Can you work these out from the model? Positions are in its coordinate system, mm. A direction names the side the tool comes from. Give positions to 0.01 mm unless a question says otherwise; leave off trailing zeros. Write each loop counter-clockwise with the first axis right and the second up, starting at its lowest first coordinate (ties: lowest second). Pieces come first, ordered by that corner, then holes. Notation, with made-up numbers: (80.25, 52) -> (91.25, 52) arc R23 cw to (91.25, 62) -> close; hole circle Ø6 at (32, 4). An arc over 180 degrees is marked (long way). Answer as CSV lines item,"result". Start each with the question number.
1. On a 3-axis mill with a long thin cutter (end or side, diameter ignored), from which of +Z, -Z, +X, -X, +Y, -Y can I reach the whole of each face in a straight line? I mean faces 1 (the face through (-3.6, 13.1, -0.5)), 2 (the face through (3.6, 13, -0.5)), 3 (the face through (4.832, 3.719, 15.463)), 4 (the face through (0.1, 18.1, -0.5)). Say none if no direction works.
2. I'm going to push flat-ended pins straight in: P1, Ø1.3, axis at x = 1, y = 17.5, coming from the +Z side; P2, Ø0.5, axis at y = 13, z = -0.5, coming from the +X side; P3, Ø8.5, axis at x = 1.5, z = 15, coming from the +Y side. Where does each tip first touch, or does it pass through?
3. If we section it at A-A on y = 27: Write out the boundary of the cut face in (x, z).
4. If we section it at C-C on z = 2: Write out the boundary of the cut face in (x, y).
5. I need wall thicknesses on line 1 (X direction, y = 2.4, z = 18); line 2 (X direction, y = 6, z = 12); line 3 (Y direction, x = 0, z = 3.35). Which ranges of each line are inside material? Lowest first, please. Write a range as [from, to].
6. If we mould it in two halves opening along Z, with no side actions, what happens to faces 5 (the face through (-0.105, 3.025, 23.095)), 6 (the face through (0, 11.4, -0.5)), 7 (the face through (-0.1, 3.5, 22.5)), 8 (the face through (1.886, 2.028, 20.46))? For each: pulls with the +Z half, pulls with the -Z half, needs draft (parallel to the pull), parting line crosses it, or undercut.
7. If we section it at B-B on x = 0: Count the separate pieces of the cut face and the enclosed holes in it, plus the area to 3 significant figures.
8. If we section it at D-D on y = 15: Write out the boundary of the cut face in (x, z).
Autodesk Inventor part; units mm, degrees
ref_plane "SD6_50_1_XY" through (-10, 15, 4.5) normal (0, 0, 1) x (1, 0, 0)
ref_plane "SD6_50_1_YZ" through (-10, 15, 4.5) normal (1, 0, 0) x (0, 1, 0)
ref_plane "SD6_50_1_ZX" through (-10, 15, 4.5) normal (0, 1, 0) x (0, 0, 1)
sketch "Sketch_15" plane through (0, 0, 0) normal (1, 0, 0) x (0, 1, 0)
  line L0 (0, 30) -> (0, 0)
  line L1 (0, 0) -> (30, 0)
  line L2 (30, 0) -> (30, 4.0858)
  arc A0 (30, 4.0858) -> (29.7071, 4.7929) centre (29, 4.0858) ccw
  line L3 (29.7071, 4.7929) -> (4.7929, 29.7071)
  arc A1 (4.7929, 29.7071) -> (4.0858, 30) centre (4.0858, 29) ccw
  line L4 (4.0858, 30) -> (0, 30)
extrude "Extrusion1" add sketch "Sketch_15" along normal mid plane 20
sketch "Sketch_16" plane through (0, 0, 0) normal (1, 0, 0) x (0, 1, 0)
  line L0 (2.9278, 34.5) -> (4.4738, 5)
  line L1 (4.4738, 5) -> (34.5, 5)
  line L2 (34.5, 5) -> (34.5, 34.5)
  line L3 (34.5, 34.5) -> (2.9278, 34.5)
extrude "Extrusion2" cut sketch "Sketch_16" along normal mid plane 15
sketch "Sketch_82" plane through (0, 0, 0) normal (1, 0, 0) x (0, 1, 0)
  line L0 (2.4278, 34.5) -> (4, 4.5)
  line L1 (4, 4.5) -> (34, 4.5)
  line L2 (34, 4.5) -> (34, 34.5)
  line L3 (34, 34.5) -> (2.4278, 34.5)
extrude "Extrusion3" cut sketch "Sketch_82" along normal mid plane 15
sketch "Sketch_17" plane through (0, 4.5, 0) normal (0, 1, 0) x (1, 0, 0)
  line L0 (-5.4209, -10.5) -> (-4.4687, -18.5299)
  arc A0 (-4.4687, -18.5299) -> (4.4687, -18.5299) centre (0, -18) ccw
  line L1 (4.4687, -18.5299) -> (5.4209, -10.5)
  line L2 (5.4209, -10.5) -> (-5.4209, -10.5)
extrude "Extrusion4" add sketch "Sketch_17" against normal blind 2.25
sketch "Sketch5" plane through (10, 0, 0) normal (0, 0, -1) x (-1, 0, 0)
  point P0 (10, 15)
hole "Hole1" at (0, 15, 0) direction (0, 0, 1) diameter 6.2 depth 5.5
sketch "Sketch6" plane through (-10, 0, 30) normal (0, -1, 0) x (1, 0, 0)
  point P0 (10, -12)
hole "Hole2" at (0, 0, 18) direction (0, 1, 0) diameter 6.2 depth 4.5
sketch "Sketch_1" plane through (0, 0, 0) normal (0, 1, 0) x (-1, 0, 0)
  line L0 (10, 0) -> (10, 30)
  line L1 (10, 30) -> (-10, 30)
  line L2 (-10, 30) -> (-10, 0)
  line L3 (-10, 0) -> (10, 0)
extrude "Extrusion5" add sketch "Sketch_1" against normal blind 1
sketch "Sketch_4" plane through (0, 0, 0) normal (0, 1, 0) x (-1, 0, 0)
  line L0 (10, 0) -> (10, 30)
  line L1 (10, 30) -> (-10, 30)
  line L2 (-10, 30) -> (-10, 0)
  line L3 (-10, 0) -> (10, 0)
extrude "Extrusion6" cut sketch "Sketch_4" against normal blind 1
sketch "Sketch_72" plane through (0, 0, 0) normal (0, 0, 1) x (1, 0, 0)
  line L0 (-3.6, 14.5) -> (-3.6, 11.6)
  arc A0 (-3.6, 11.6) -> (-3.4, 11.4) centre (-3.4, 11.6) ccw
  line L1 (-3.4, 11.4) -> (3.4, 11.4)
  arc A1 (3.4, 11.4) -> (3.6, 11.6) centre (3.4, 11.6) ccw
  line L2 (3.6, 11.6) -> (3.6, 14.5)
  line L3 (3.6, 14.5) -> (3.0594, 14.5)
  arc A2 (-3.0594, 14.5) -> (3.0594, 14.5) centre (0, 15) ccw
  line L4 (-3.0594, 14.5) -> (-3.6, 14.5)
extrude "Extrusion7" add sketch "Sketch_72" against normal blind 1
sketch "Sketch_73" plane through (0, 0, 0) normal (0, 0, 1) x (1, 0, 0)
  line L0 (-3.6, 15.5) -> (-3.0594, 15.5)
  arc A0 (3.0594, 15.5) -> (-3.0594, 15.5) centre (0, 15) ccw
  line L1 (3.0594, 15.5) -> (3.6, 15.5)
  line L2 (3.6, 15.5) -> (3.6, 18.4)
  arc A1 (3.6, 18.4) -> (3.4, 18.6) centre (3.4, 18.4) ccw
  line L3 (3.4, 18.6) -> (-3.4, 18.6)
  arc A2 (-3.4, 18.6) -> (-3.6, 18.4) centre (-3.4, 18.4) ccw
  line L4 (-3.6, 18.4) -> (-3.6, 15.5)
extrude "Extrusion8" add sketch "Sketch_73" against normal blind 1
sketch "Sketch_86" plane through (0, 4.5, 0) normal (0, 1, 0) x (1, 0, 0)
  line L0 (-5.4209, -10.5) -> (-4.4687, -18.5299)
  arc A0 (-4.4687, -18.5299) -> (4.4687, -18.5299) centre (0, -18) ccw
  line L1 (4.4687, -18.5299) -> (5.4209, -10.5)
  line L2 (5.4209, -10.5) -> (-5.4209, -10.5)
extrude "Extrusion9" cut sketch "Sketch_86" against normal blind 0.5
ref_plane "SD6_50_1_XY" through (-10, 15, 4.5) normal (0, 0, 1) x (1, 0, 0)
ref_plane "SD6_50_1_YZ" through (-10, 15, 4.5) normal (1, 0, 0) x (0, 1, 0)
ref_plane "SD6_50_1_ZX" through (-10, 15, 4.5) normal (0, 1, 0) x (0, 0, 1)
ref_plane "SD6_50_2_XY" through (10, 15, 4.5) normal (0, 0, 1) x (1, 0, 0)
ref_plane "SD6_50_2_YZ" through (10, 15, 4.5) normal (1, 0, 0) x (0, 1, 0)
ref_plane "SD6_50_2_ZX" through (10, 15, 4.5) normal (0, 1, 0) x (0, 0, 1)
ref_plane "SD6_50_3_XY" through (-10, 4.5, 18) normal (0, 1, 0) x (1, 0, 0)
ref_plane "SD6_50_3_YZ" through (-10, 4.5, 18) normal (1, 0, 0) x (0, 0, -1)
ref_plane "SD6_50_3_ZX" through (-10, 4.5, 18) normal (0, 0, -1) x (0, 1, 0)
ref_plane "SD6_50_4_XY" through (10, 4.5, 18) normal (0, 1, 0) x (1, 0, 0)
ref_plane "SD6_50_4_YZ" through (10, 4.5, 18) normal (1, 0, 0) x (0, 0, -1)
ref_plane "SD6_50_4_ZX" through (10, 4.5, 18) normal (0, 0, -1) x (0, 1, 0)
ref_plane "a10_to_bolt_XY" through (15, 15, 4.5) normal (0, 0, 1) x (1, 0, 0)
ref_plane "a10_to_bolt_YZ" through (15, 15, 4.5) normal (1, 0, 0) x (0, 1, 0)
ref_plane "a10_to_bolt_ZX" through (15, 15, 4.5) normal (0, 1, 0) x (0, 0, 1)
ref_plane "a11_to_bolt_XY" through (-15, 4.5, 18) normal (0, 1, 0) x (1, 0, 0)
ref_plane "a11_to_bolt_YZ" through (-15, 4.5, 18) normal (1, 0, 0) x (0, 0, -1)
ref_plane "a11_to_bolt_ZX" through (-15, 4.5, 18) normal (0, 0, -1) x (0, 1, 0)
ref_plane "a12_to_bolt_XY" through (15, 4.5, 18) normal (0, 1, 0) x (1, 0, 0)
ref_plane "a12_to_bolt_YZ" through (15, 4.5, 18) normal (1, 0, 0) x (0, 0, -1)
ref_plane "a12_to_bolt_ZX" through (15, 4.5, 18) normal (0, 0, -1) x (0, 1, 0)
ref_plane "a13_to_bolt_XY" through (0, 4.5, 38) normal (0, 1, 0) x (1, 0, 0)
ref_plane "a13_to_bolt_YZ" through (0, 4.5, 38) normal (1, 0, 0) x (0, 0, -1)
ref_plane "a13_to_bolt_ZX" through (0, 4.5, 38) normal (0, 0, -1) x (0, 1, 0)
ref_plane "a14_to_bolt_XY" through (0, 30, 4.5) normal (0, 0, 1) x (1, 0, 0)
ref_plane "a14_to_bolt_YZ" through (0, 30, 4.5) normal (1, 0, 0) x (0, 1, 0)
ref_plane "a14_to_bolt_ZX" through (0, 30, 4.5) normal (0, 1, 0) x (0, 0, 1)
ref_plane "a1_to_bolt_XY" through (-10, 20, 4.5) normal (0, 0, 1) x (1, 0, 0)
ref_plane "a1_to_bolt_YZ" through (-10, 20, 4.5) normal (1, 0, 0) x (0, 1, 0)
ref_plane "a1_to_bolt_ZX" through (-10, 20, 4.5) normal (0, 1, 0) x (0, 0, 1)
ref_plane "a2_to_bolt_XY" through (-10, 4.5, 15) normal (0, 1, 0) x (1, 0, 0)
ref_plane "a2_to_bolt_YZ" through (-10, 4.5, 15) normal (1, 0, 0) x (0, 0, -1)
ref_plane "a2_to_bolt_ZX" through (-10, 4.5, 15) normal (0, 0, -1) x (0, 1, 0)
ref_plane "a3_to_bolt_XY" through (1, 15, 4.5) normal (0, 0, 1) x (1, 0, 0)
ref_plane "a3_to_bolt_YZ" through (1, 15, 4.5) normal (1, 0, 0) x (0, 1, 0)
ref_plane "a3_to_bolt_ZX" through (1, 15, 4.5) normal (0, 1, 0) x (0, 0, 1)
ref_plane "a4_to_bolt_XY" through (1, 4, 18) normal (0, 1, 0) x (1, 0, 0)
ref_plane "a4_to_bolt_YZ" through (1, 4, 18) normal (1, 0, 0) x (0, 0, -1)
ref_plane "a4_to_bolt_ZX" through (1, 4, 18) normal (0, 0, -1) x (0, 1, 0)
ref_plane "a55_to_bolt_XY" through (0, 18, 4.5) normal (0, 0, 1) x (1, 0, 0)
ref_plane "a55_to_bolt_YZ" through (0, 18, 4.5) normal (1, 0, 0) x (0, 1, 0)
ref_plane "a55_to_bolt_ZX" through (0, 18, 4.5) normal (0, 1, 0) x (0, 0, 1)
ref_plane "a5_to_bolt_XY" through (0, 15, 4.5) normal (0, 0, 1) x (1, 0, 0)
ref_plane "a5_to_bolt_YZ" through (0, 15, 4.5) normal (1, 0, 0) x (0, 1, 0)
ref_plane "a5_to_bolt_ZX" through (0, 15, 4.5) normal (0, 1, 0) x (0, 0, 1)
ref_plane "a6_to_bolt_XY" through (0, 4, 18) normal (0, 1, 0) x (1, 0, 0)
ref_plane "a6_to_bolt_YZ" through (0, 4, 18) normal (1, 0, 0) x (0, 0, -1)
ref_plane "a6_to_bolt_ZX" through (0, 4, 18) normal (0, 0, -1) x (0, 1, 0)
ref_plane "a7_to_bolt_XY" through (0, 35, 4.5) normal (0, 0, 1) x (1, 0, 0)
ref_plane "a7_to_bolt_YZ" through (0, 35, 4.5) normal (1, 0, 0) x (0, 1, 0)
ref_plane "a7_to_bolt_ZX" through (0, 35, 4.5) normal (0, 1, 0) x (0, 0, 1)
ref_plane "a8_to_bolt_XY" through (0, 4.5, 48) normal (0, 1, 0) x (1, 0, 0)
ref_plane "a8_to_bolt_YZ" through (0, 4.5, 48) normal (1, 0, 0) x (0, 0, -1)
ref_plane "a8_to_bolt_ZX" through (0, 4.5, 48) normal (0, 0, -1) x (0, 1, 0)
ref_plane "a9_to_bolt_XY" through (-15, 15, 4.5) normal (0, 0, 1) x (1, 0, 0)
ref_plane "a9_to_bolt_YZ" through (-15, 15, 4.5) normal (1, 0, 0) x (0, 1, 0)
ref_plane "a9_to_bolt_ZX" through (-15, 15, 4.5) normal (0, 1, 0) x (0, 0, 1)
ref_plane "bracket_to_dummy_XY" through (0, 0, 0) normal (0, 1, 0) x (1, 0, 0)
ref_plane "bracket_to_dummy_YZ" through (0, 0, 0) normal (1, 0, 0) x (0, 0, -1)
ref_plane "bracket_to_dummy_ZX" through (0, 0, 0) normal (0, 0, -1) x (0, 1, 0)
ref_plane "hole_x1_bolt_XY" through (-10, 35, 4.5) normal (0, 0, 1) x (1, 0, 0)
ref_plane "hole_x1_bolt_YZ" through (-10, 35, 4.5) normal (1, 0, 0) x (0, 1, 0)
ref_plane "hole_x1_bolt_ZX" through (-10, 35, 4.5) normal (0, 1, 0) x (0, 0, 1)
ref_plane "holex2_to_bolt_XY" through (10, 35, 4.5) normal (0, 0, 1) x (1, 0, 0)
ref_plane "holex2_to_bolt_YZ" through (10, 35, 4.5) normal (1, 0, 0) x (0, 1, 0)
ref_plane "holex2_to_bolt_ZX" through (10, 35, 4.5) normal (0, 1, 0) x (0, 0, 1)
ref_plane "holex3_to_bolt_XY" through (10, 4.5, 35) normal (0, 1, 0) x (1, 0, 0)
ref_plane "holex3_to_bolt_YZ" through (10, 4.5, 35) normal (1, 0, 0) x (0, 0, -1)
ref_plane "holex3_to_bolt_ZX" through (10, 4.5, 35) normal (0, 0, -1) x (0, 1, 0)
ref_plane "holex4_to_bolt_XY" through (10, 4.5, 15) normal (0, 1, 0) x (1, 0, 0)
ref_plane "holex4_to_bolt_YZ" through (10, 4.5, 15) normal (1, 0, 0) x (0, 0, -1)
ref_plane "holex4_to_bolt_ZX" through (10, 4.5, 15) normal (0, 0, -1) x (0, 1, 0)
ref_plane "holex5_to_bolt_XY" through (-10, 4.5, 35) normal (0, 1, 0) x (1, 0, 0)
ref_plane "holex5_to_bolt_YZ" through (-10, 4.5, 35) normal (1, 0, 0) x (0, 0, -1)
ref_plane "holex5_to_bolt_ZX" through (-10, 4.5, 35) normal (0, 0, -1) x (0, 1, 0)
ref_plane "holex6_to_bolt_XY" through (10, 20, 4.5) normal (0, 0, 1) x (1, 0, 0)
ref_plane "holex6_to_bolt_YZ" through (10, 20, 4.5) normal (1, 0, 0) x (0, 1, 0)
ref_plane "holex6_to_bolt_ZX" through (10, 20, 4.5) normal (0, 1, 0) x (0, 0, 1)
properties part number "HBLFSNE6_"
Computed values:
1,face 1,"-Z, -X, +Y, -Y"
1,face 2,"-Z, +X, +Y, -Y"
1,face 3,"+Z, +Y"
1,face 4,"+Z, -Z"
2,P1,"stops at z = 4.5"
2,P2,"stops at x = 3.6"
2,P3,"stops at y = 4"
3,outline,"(-10, 0) -> (10, 0) -> (10, 7.5) -> (7.5, 7.5) -> (7.5, 4.5) -> (-7.5, 4.5) -> (-7.5, 7.5) -> (-10, 7.5) -> close"
4,outline,"(-10, 0) -> (10, 0) -> (10, 30) -> (-10, 30) -> close; hole circle Ø6.2 at (0, 15)"
5,line 1,"x = [-10, -3.1], [3.1, 10]"
5,line 2,"x = [-10, -7.5], [7.5, 10]"
5,line 3,"y = [0, 11.9], [18.1, 30]"
6,face 5,"undercut"
6,face 6,"needs draft"
6,face 7,"pulls with the +Z half"
6,face 8,"undercut"
7,separate pieces,"3"
7,enclosed holes,"0"
7,area,"176 mm2"
8,outline,"(-10, 0) -> (-3.1, 0) -> (-3.1, 4.5) -> (-7.5, 4.5) -> (-7.5, 19.5) -> (-10, 19.5) -> close; (3.1, 0) -> (10, 0) -> (10, 19.5) -> (7.5, 19.5) -> (7.5, 4.5) -> (3.1, 4.5) -> close"
